Design review of the part built by this model. Coordinates are the model's own, in mm. Round coordinates to 2 decimals unless told otherwise and drop trailing zeros. Loops run counter-clockwise (first coordinate to the right, second up) from the corner with the lowest first, then second, coordinate; pieces in that order, holes last. Notation, with made-up numbers: M 87,22.5 L 118,22.5 A13 cw 118,33.5 Z; hole C 67.25,50 d8. An arc over 180 degrees is marked long. One line per item, written item: value. Start each with the question number.
Item 1: We need section C-C (y = 73). Write out the cut boundary in (x, z), then the cut area to 3 significant figures.
Item 2: For line 1 along X through (y, z) = (295.5, -580); line 2 along Z through (x, y) = (85, 292); line 3 along Z through (x, y) = (-100, 291), list the stretches that pass through material, from the lowest coordinate up.
Item 3: We need section B-B (z = -308.5). Write out the cut boundary in (x, y), then the cut area to 3 significant figures.
Item 4: Clearance check with flat-ended pins moving along their axes: pin 1 (21 mm diameter, centred on x = -85, z = 1250, fed in from +Y); pin 2 (3 mm diameter, centred on y = 165.5, z = 685.5, fed in from -X). State where each tip first meets the part, or that it passes through.
Item 5: We need section A-A (x = -46). Write out the cut boundary in (y, z).
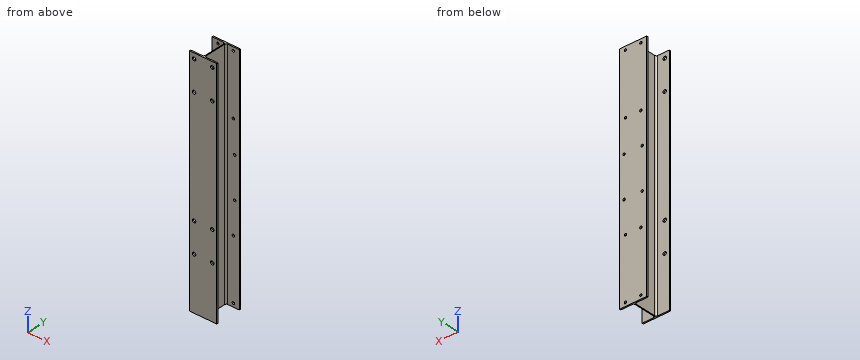
from build123d import *

# Parameters (mm, degrees)
EXTRUDE_1_DEPTH     = 1290
SKETCH_2_R          = 19
CUT_EXTRUDE_1_DEPTH = 60
SKETCH_3_R          = 13
CUT_EXTRUDE_2_DEPTH = 60


with BuildPart() as part:
    # Эскиз1 → Бобышка-Вытянуть1 (new body, symmetric)
    with BuildSketch(Plane.XY):
        with BuildLine():
            Line((150, 300), (-150, 300))
            Line((-150, 300), (-150, 285))
            Line((-150, 285), (-23, 285))
            ThreePointArc((-23, 285), (-10.272077939, 279.727922061), (-5, 267))
            Line((-5, 267), (-5, 33))
            ThreePointArc((-5, 33), (-10.272077939, 20.272077939), (-23, 15))
            Line((-23, 15), (-150, 15))
            Line((-150, 15), (-150, 0))
            Line((-150, 0), (150, 0))
            Line((150, 0), (150, 15))
            Line((150, 15), (23, 15))
            ThreePointArc((23, 15), (10.272077939, 20.272077939), (5, 33))
            Line((5, 33), (5, 267))
            ThreePointArc((5, 267), (10.272077939, 279.727922061), (23, 285))
            Line((23, 285), (150, 285))
            Line((150, 285), (150, 300))
        make_face()
    extrude(amount=EXTRUDE_1_DEPTH, both=True)

    # Эскиз2 → Вырез-Вытянуть1 (cut)
    with BuildSketch(Plane.XZ):
        with Locations((-100, 1230)):
            Circle(SKETCH_2_R)
        with Locations((100, 1230)):
            Circle(SKETCH_2_R)
        with Locations((-100, 900)):
            Circle(SKETCH_2_R)
        with Locations((100, 900)):
            Circle(SKETCH_2_R)
        with Locations((-100, -705)):
            Circle(SKETCH_2_R)
        with Locations((100, -705)):
            Circle(SKETCH_2_R)
        with Locations((-100, -375)):
            Circle(SKETCH_2_R)
        with Locations((100, -375)):
            Circle(SKETCH_2_R)
    extrude(amount=-CUT_EXTRUDE_1_DEPTH, mode=Mode.SUBTRACT)

    # Эскиз3 → Вырез-Вытянуть2 (cut)
    with BuildSketch(Plane(origin=(0, 300, 0), x_dir=(1, 0, 0), z_dir=(0, 1, 0))):
        with Locations((-85, -1250)):
            Circle(SKETCH_3_R)
        with Locations((85, -1250)):
            Circle(SKETCH_3_R)
        with Locations((-85, -580)):
            Circle(SKETCH_3_R)
        with Locations((85, -580)):
            Circle(SKETCH_3_R)
        with Locations((-100, -225)):
            Circle(SKETCH_3_R)
        with Locations((100, -225)):
            Circle(SKETCH_3_R)
        with Locations((-100, 225)):
            Circle(SKETCH_3_R)
        with Locations((100, 225)):
            Circle(SKETCH_3_R)
        with Locations((-85, 580)):
            Circle(SKETCH_3_R)
        with Locations((85, 580)):
            Circle(SKETCH_3_R)
        with Locations((-85, 1250)):
            Circle(SKETCH_3_R)
        with Locations((85, 1250)):
            Circle(SKETCH_3_R)
    extrude(amount=-CUT_EXTRUDE_2_DEPTH, mode=Mode.SUBTRACT)


solid = part.part
A:
1. outline: M -5,-1290 L 5,-1290 L 5,1290 L -5,1290 Z
1. area: 25,800 mm2
2. line 1: -150 to -98, -72 to 72, 98 to 150
2. line 2: -1290 to -1263, -1237 to -593, -567 to 567, 593 to 1237, 1263 to 1290
2. line 3: -1290 to -238, -212 to 212, 238 to 1290
3. outline: M -150,0 L 150,0 L 150,15 L 23,15 A18 cw 5,33 L 5,267 A18 cw 23,285 L 150,285 L 150,300 L -150,300 L -150,285 L -23,285 A18 cw -5,267 L -5,33 A18 cw -23,15 L -150,15 Z
3. area: 12,000 mm2
4. pin 1: y = 15
4. pin 2: x = -5
5. outline: M 0,-1290 L 15,-1290 L 15,1290 L 0,1290 Z; M 285,-1290 L 300,-1290 L 300,1290 L 285,1290 Z
